Geometry check sheet. Reference: drawing and pictorial views, mm from the part's lowest x, y, z. Coordinates: 2 decimals unless noted, no trailing zeros. Loops run counter-clockwise (first coordinate to the right, second up) from the corner with the lowest first, then second, coordinate; pieces in that order, holes last. Notation, with made-up numbers: (4.25, -0.75) -> (31.25, -0.75) arc R14 ccw to (31.25, 17.25) -> close; hole circle Ø8 at (-3, -24). An arc over 180 degrees is marked (long way). Use CSV: the item, a comma, the result in double quotes.
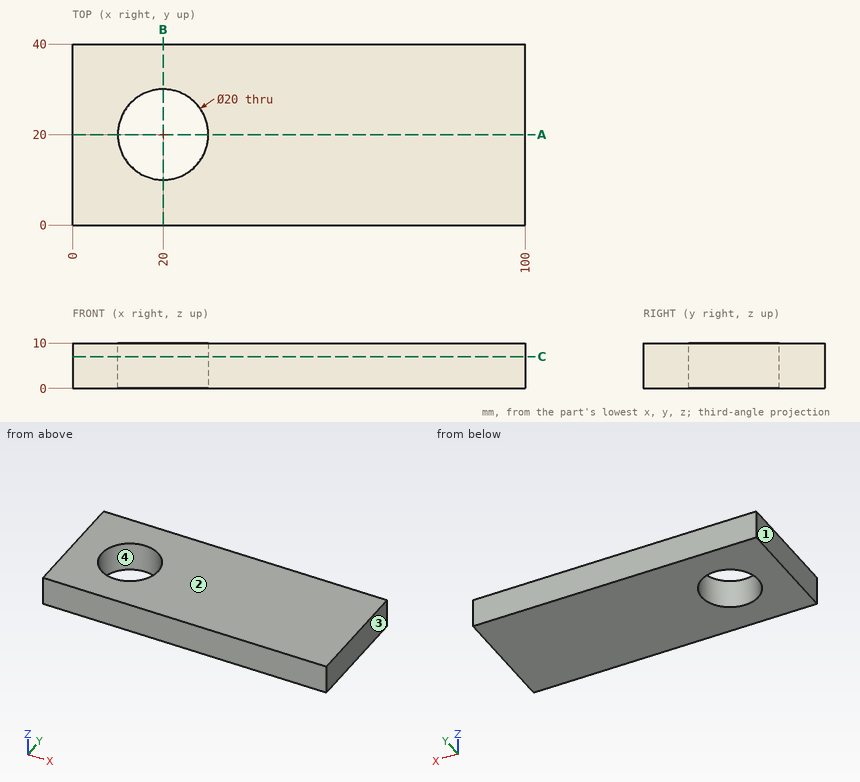
1) Draft check along X on the marked faces 1, 2, 3 and 4. Enter one of: released by +X, released by -X, zero draft, split by the parting line, or undercut.
Answer below:
face 1,"released by -X"
face 2,"zero draft"
face 3,"released by +X"
face 4,"undercut"
2) Thickness scan on line 1 along Y through (x, z) = (20, 3.75); line 2 along Y through (x, z) = (16, 9); line 3 along X through (y, z) = (21.5, 2). Record the ranges inside material, lowest first. Write a range as from..to.
Answer below:
line 1,"y = 0..10, 30..40"
line 2,"y = 0..10.83, 29.17..40"
line 3,"x = 0..10.11, 29.89..100"
3) Cross-section at A-A on y = 20. Record the boundary of the cut face in (x, z), and give its area (3 significant figures).
Answer below:
outline,"(0, 0) -> (10, 0) -> (10, 10) -> (0, 10) -> close; (30, 0) -> (100, 0) -> (100, 10) -> (30, 10) -> close"
area,"800 mm²"
4) Cross-section at B-B on x = 20. Record the boundary of the cut face in (y, z), and give its area (3 significant figures).
Answer below:
outline,"(0, 0) -> (10, 0) -> (10, 10) -> (0, 10) -> close; (30, 0) -> (40, 0) -> (40, 10) -> (30, 10) -> close"
area,"200 mm²"
5) Cross-section at C-C on z = 7. Record the boundary of the cut face in (x, y), and give its area (3 significant figures).
Answer below:
outline,"(0, 0) -> (100, 0) -> (100, 40) -> (0, 40) -> close; hole circle Ø20 at (20, 20)"
area,"3,690 mm²"
